from build123d import *

# Parameters (mm, degrees)
SKETCH_1_W         = 50
SKETCH_1_H         = 40
SKETCH_1_R         = 2.1
EXTRUDE_590_DEPTH  = 4
SKETCH_2_W         = 34
SKETCH_2_H         = 14
SKETCH_2_H_2       = 8
SKETCH_2_R         = 2.1
EXTRUDE_1234_DEPTH = 4
FILLET_3_R         = 3
FILLET_5_R         = 5


with BuildPart() as part:
    # 草图1 → Extrude 590 (new body)
    with BuildSketch(Plane(origin=(0, 0, 0), x_dir=(1, 0, 0), z_dir=(0, 1, 0))):
        with Locations((-15, -10)):
            Rectangle(SKETCH_1_W, SKETCH_1_H)
        Circle(SKETCH_1_R, mode=Mode.SUBTRACT)
        with BuildLine():
            ThreePointArc((-24.718674601, 4.358569259), (-23.586284782, -8.584705597), (-16.133969003, -19.227715522))
            ThreePointArc((-16.133969003, -19.227715522), (-12.471005666, -18.907247755), (-12.791473433, -15.244284418))
            ThreePointArc((-12.791473433, -15.244284418), (-18.699883154, -6.806200852), (-19.597674285, 3.455598736))
            ThreePointArc((-19.597674285, 3.455598736), (-21.706689181, 6.467584155), (-24.718674601, 4.358569259))
        make_face(mode=Mode.SUBTRACT)
    extrude(amount=EXTRUDE_590_DEPTH)

    # 草图2 → Extrude 1234 (add, through all)
    with BuildSketch(Plane(origin=(0, 4, 0), x_dir=(1, 0, 0), z_dir=(0, 1, 0))):
        with Locations((-15, 17)):
            Rectangle(SKETCH_2_W, SKETCH_2_H)
        with Locations((-15, 28)):
            Rectangle(SKETCH_2_W, SKETCH_2_H_2)
        with Locations((-3, 28)):
            Circle(SKETCH_2_R, mode=Mode.SUBTRACT)
        with Locations((-27, 28)):
            Circle(SKETCH_2_R, mode=Mode.SUBTRACT)
    extrude(amount=-EXTRUDE_1234_DEPTH)

    # 圆角3
    fillet_3_edges = [part.edges().sort_by_distance(p)[0] for p in [
        (2, 2, -10),
        (-32, 2, -10),
        (-40, 2, -10),
        (10, 2, -10),
    ]]
    fillet(fillet_3_edges, radius=FILLET_3_R)

    # 圆角5
    fillet_5_edges = [part.edges().sort_by_distance(p)[0] for p in [
        (2, 2, -32),
        (-32, 2, -32),
        (10, 2, 30),
        (-40, 2, 30),
    ]]
    fillet(fillet_5_edges, radius=FILLET_5_R)


solid = part.part
Model file for the job. Use its own axes, mm. A direction names the side the tool comes from. Round coordinates to 2 decimals unless told otherwise and drop trailing zeros. Order: outer loops, then holes, each group sorted by start corner. A loop starts at its lowest first (then second) coordinate and runs counter-clockwise, first axis right, second up.
(1) Drill centre lines: line 1 (X direction, y = 3.1, z = -1.5); line 2 (X direction, y = 1.5, z = -28.5); line 3 (X direction, y = 0.4, z = -5). Where is each one in solid material? Low to high.
(2) 3-axis set-ups, long thin cutter, end or side, ignore diameter. For faces 5 (the face through (-23.65, 1.97, 8.41)), 6 (the face through (6, 2, -10)), 7 (the face through (-32.9, 1.97, -10.86)): which of +Z, -Z, +X, -X, +Y, -Y reach the whole face in a straight line?
(3) Band-saw the part on A-A (x = 0). List the corners of the cut face in (y, z), then the cut area to 3 significant figures.
(4) Pin check, flat tips, straight feed: pin 1 (1.2 mm diameter, centred on y = 1, z = -18, fed in from +X); pin 2 (1.6 mm diameter, centred on x = -36, y = 1.5, fed in from -Z). Stop position of each tip, or through.
(5) Pull direction Z, two halves, no side cores. Call faces 1 (the face through (-21.65, 1.972, -6.457)), 2 (the face through (-18.65, 1.97, 6.94)), 3 (the face through (10, 2, 9)), 4 (the face through (-31, 2, -30)): released by +Z, released by -Z, zero draft, split by the parting line, or undercut.
(6) Band-saw the part on B-B (z = 0). List the corners of the cut face in (x, y), then the cut area to 3 significant figures.
(7) Band-saw the part on D-D (y = 3.3). List the corners of the cut face in (x, z).
(8) Band-saw the part on C-C (z = 14.5). List the corners of the cut face in (x, y), then the cut area to 3 significant figures.
Verdict:
1. line 1: x = -40 to -25.06, -19.84 to -1.47, 1.47 to 10
1. line 2: x = -31.77 to -29.04, -24.96 to -5.04, -0.96 to 1.77
1. line 3: x = -40 to -24.52, -19.8 to 10
2. face 5: +Y, -Y
2. face 6: -Z, +X, +Y, -Y
2. face 7: -Z, -X, +Y, -Y
3. outline: (0, -31) - (4, -31) - (4, -2.1) - (0, -2.1) - close; (0, 2.1) - (4, 2.1) - (4, 30) - (0, 30) - close
3. area: 227 mm2
4. pin 1: stops at x = 2
4. pin 2: stops at z = -10
5. face 1: undercut
5. face 2: undercut
5. face 3: zero draft
5. face 4: released by -Z
6. outline: (-40, 0) - (-25.1, 0) - (-25.1, 4) - (-40, 4) - close; (-19.9, 0) - (-2.1, 0) - (-2.1, 4) - (-19.9, 4) - close; (2.1, 0) - (10, 0) - (10, 4) - (2.1, 4) - close
6. area: 162 mm2
7. outline: (-40, -7) arc R3 ccw to (-37, -10) - (-35, -10) arc R3 cw to (-32, -13) - (-32, -27) arc R5 ccw to (-27, -32) - (-3, -32) arc R5 ccw to (2, -27) - (2, -13) arc R3 cw to (5, -10) - (7, -10) arc R3 ccw to (10, -7) - (10, 25) arc R5 ccw to (5, 30) - (-35, 30) arc R5 ccw to (-40, 25) - close; hole circle Ø4.2 at (-27, -28); hole (-24.72, -4.36) arc R2.6 ccw to (-19.6, -3.46) arc R19.9 cw to (-12.79, 15.24) arc R2.6 ccw to (-16.13, 19.23) arc R25.1 ccw to start; hole circle Ø4.2 at (-3, -28); hole circle Ø4.2 at (0, 0)
8. outline: (-40, 0) - (-20.49, 0) - (-20.49, 4) - (-40, 4) - close; (-13.63, 0) - (10, 0) - (10, 4) - (-13.63, 4) - close
8. area: 173 mm2
